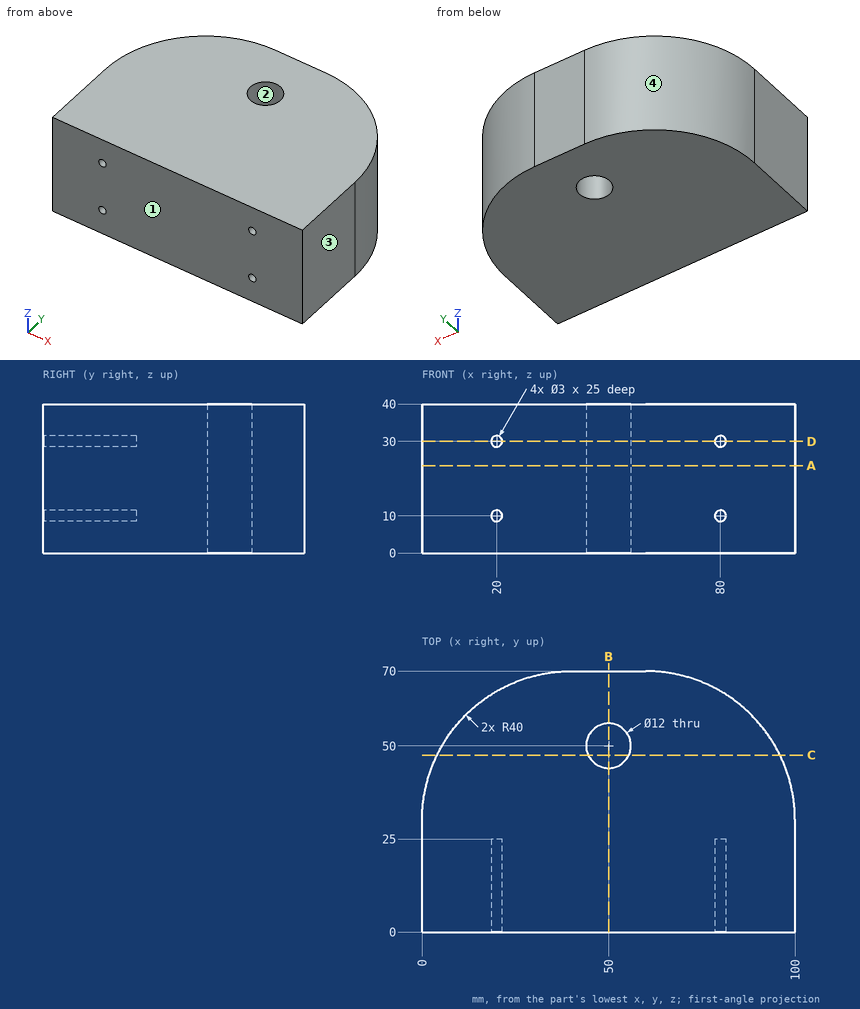
Here's the drawing with two shaded views (mm, measured from the low corner). I have some questions. Give positions to 0.01 mm unless a question says otherwise; leave off trailing zeros. Loops run counter-clockwise (first coordinate to the right, second up) from the corner with the lowest first, then second, coordinate; pieces in that order, holes last. Notation, with made-up numbers: (-12, 40) - (-3, 40) arc R26 ccw to (-3, 67) - close; hole circle Ø11 at (3.5, -28.5). An arc over 180 degrees is marked (long way). Answer in a Markdown table with one row per item. Add a question column.
Q1. If we section it at B-B (x = 50): List the corners of the cut face in (y, z) for me.
Q2. For pin 1 (2.5 mm diameter, centred on x = 20, z = 30, fed in from +Y); pin 2 (1.5 mm diameter, centred on y = 35.5, z = 31, fed in from -X); pin 3 (11 mm diameter, centred on x = 50, y = 50, fed in from -Z); pin 4 (3 mm diameter, centred on y = 55.5, z = 7.5, fed in from +X), each with a flat end and sliding along its axis, tell me the tip position at first contact or that it passes through.
Q3. We'd pull the mould along Y, two halves only. Please class the marked faces 1, 2, 3 and 4: +Y half, -Y half, draft (parallel to the pull), parting line (faces both ways), or undercut.
Q4. If we section it at D-D (z = 30): List the corners of the cut face in (x, y) for me.
Q5. Please list where these lines run through material, in increasing order: L1, parallel to Z at x = 80, y = 15.25; L2, parallel to Y at x = 50, z = 20; L3, parallel to X at y = 47, z = 37. Write a range as from..to.
Q6. If we section it at A-A (z = 23.5): List the corners of the cut face in (x, y) for me.
Q7. If we section it at C-C (y = 47.5): List the corners of the cut face in (x, z) for me, plus the area to 3 significant figures.
The answers:
| question | item | result |
|---|---|---|
| 1 | outline | (0, 0) - (44, 0) - (44, 40) - (0, 40) - close; (56, 0) - (70, 0) - (70, 40) - (56, 40) - close |
| 2 | pin 1 | stops at y = 65.33 |
| 2 | pin 2 | stops at x = 0.28 |
| 2 | pin 3 | passes through |
| 2 | pin 4 | stops at x = 92 |
| 3 | face 1 | -Y half |
| 3 | face 2 | undercut |
| 3 | face 3 | draft |
| 3 | face 4 | +Y half |
| 4 | outline | (0, 0) - (18.5, 0) - (18.5, 25) - (21.5, 25) - (21.5, 0) - (78.5, 0) - (78.5, 25) - (81.5, 25) - (81.5, 0) - (100, 0) - (100, 30) arc R40 ccw to (60, 70) - (40, 70) arc R40 ccw to (0, 30) - close; hole circle Ø12 at (50, 50) |
| 5 | L1 | z = 0..8.5, 11.5..28.5, 31.5..40 |
| 5 | L2 | y = 0..44, 56..70 |
| 5 | L3 | x = 3.79..44.8, 55.2..96.21 |
| 6 | outline | (0, 0) - (100, 0) - (100, 30) arc R40 ccw to (60, 70) - (40, 70) arc R40 ccw to (0, 30) - close; hole circle Ø12 at (50, 50) |
| 7 | outline | (4.03, 0) - (44.55, 0) - (44.55, 40) - (4.03, 40) - close; (55.45, 0) - (95.97, 0) - (95.97, 40) - (55.45, 40) - close |
| 7 | area | 3,240 mm^2 |
